The model under review builds one solid part; all positions refer to its coordinate system, in mm. Face numbers are marked on the shaded views. A direction names the side the tool comes from. Give positions to 0.01 mm unless a question says otherwise; leave off trailing zeros. Loops run counter-clockwise (first coordinate to the right, second up) from the corner with the lowest first, then second, coordinate; pieces in that order, holes last. Notation, with made-up numbers: M 61.25,45.25 L 101.25,45.25 A12 ccw 101.25,55.25 Z; hole C 13.25,22 d4. An arc over 180 degrees is marked long. Put each result on its own line as item: value. Start each with the question number.
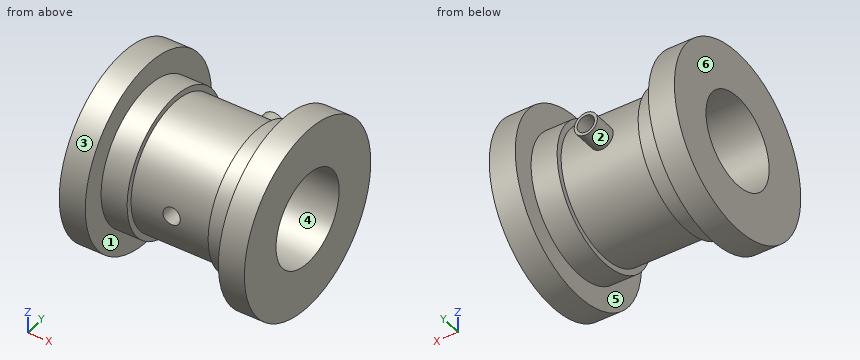
```python
from build123d import *

# Parameters (mm, degrees)
BOSS_EXTRUDE1_REACH      = 96.678
BOSS_EXTRUDE1_END_RADIUS = 22
SKETCH2_R                = 4
SKETCH3_R                = 3
CUT_EXTRUDE1_DEPTH       = 95.678403028


with BuildPart() as part:
    # Sketch1 → Revolve1 (revolve)
    with BuildSketch(Plane.XY, mode=Mode.PRIVATE) as revolve1_sk:
        Polygon((0, 16), (64, 16), (64, 32), (55, 32), (55, 24), (46, 24), (46, 22), (18, 22), (18, 24), (9, 24), (9, 32), (0, 32), align=None)
    revolve(revolve1_sk.sketch.rotate(Axis((0, 0, 0), (1, 0, 0)), 90), axis=Axis((0, 0, 0), (1, 0, 0)))

    # Boss-Extrude1: up to this cylinder (the profile starts outside it)
    boss_extrude1_end = Plane(origin=(32, 0, 0), z_dir=(-1, 0, 0)) * Cylinder(BOSS_EXTRUDE1_END_RADIUS, 238.356, mode=Mode.PRIVATE)
    # Sketch2 → Boss-Extrude1 (add, up to the surface)
    with BuildSketch(Plane(origin=(0, 30, 0), x_dir=(1, 0, 0), z_dir=(0, 1, 0)), mode=Mode.PRIVATE) as boss_extrude1_sk1:
        with Locations(Location((32, -1, 0), (0, 0, 270))):
            Circle(SKETCH2_R)
    boss_extrude1_tool1 = extrude(boss_extrude1_sk1.sketch, amount=-BOSS_EXTRUDE1_REACH, mode=Mode.PRIVATE) - boss_extrude1_end
    add(boss_extrude1_tool1.solids().sort_by_distance((32, 30, 1))[0])

    # Sketch3 → Cut-Extrude1 (cut, through all)
    with BuildSketch(Plane(origin=(0, 30, 0), x_dir=(1, 0, 0), z_dir=(0, 1, 0))):
        with Locations(Location((32, -1, 0), (0, 0, 270))):
            Circle(SKETCH3_R)
    extrude(amount=-CUT_EXTRUDE1_DEPTH, mode=Mode.SUBTRACT)


solid = part.part
```
Item 1: Clearance check with flat-ended pins moving along their axes: pin 1 Ø6.5 at (x, z) = (30.5, 0.5) entering from +Y; pin 2 Ø6 at (x, z) = (22.5, 7.5) entering from +Y; pin 3 Ø12 at (y, z) = (-6, 22) entering from -X; pin 4 Ø1.5 at (x, y) = (44, 4) entering from -Z. State where each tip first meets the part, or that it passes through.
Item 2: Consider section C-C, the plane z = -7. Write out the cut boundary in (x, y).
Item 3: To check wall thickness, follow L1, parallel to X at y = -17, z = -15; L2, parallel to X at y = 23, z = 1; L3, parallel to Z at x = 32, y = 25. State the ranges of each line that lie inside material, in increasing order. Write a range as [from, to].
Item 4: Draft analysis for pull direction X (two halves, no side actions). For the marked faces 4, 5 and 6, state which applies: +X half, -X half, draft (parallel to the pull), parting line (faces both ways), or undercut.
Item 5: Tool access review of the marked faces 1, 2 and 3: name each direction out of +Z, -Z, +X, -X, +Y, -Y from which nothing blocks a thin tool from reaching the whole face with its end or side.
Item 6: Consider section B-B, the plane x = 32. Write out the cut boundary in (y, z).
Item 7: Consider section A-A, the plane y = -11. Write out the cut boundary in (x, z), plus the area to 3 significant figures.
Item 8: Consider section D-D, the plane x = 23.5. Write out the cut boundary in (y, z).
Report:
1. pin 1: y = 30
1. pin 2: y = 21.53
1. pin 3: x = 0
1. pin 4: z = -21.76
2. outline: M 0,-31.22 L 9,-31.22 L 9,-22.96 L 18,-22.96 L 18,-20.86 L 46,-20.86 L 46,-22.96 L 55,-22.96 L 55,-31.22 L 64,-31.22 L 64,-14.39 L 0,-14.39 Z; M 0,14.39 L 64,14.39 L 64,31.22 L 55,31.22 L 55,22.96 L 46,22.96 L 46,20.86 L 18,20.86 L 18,22.96 L 9,22.96 L 9,31.22 L 0,31.22 Z
3. L1: [0, 18], [46, 64]
3. L2: [0, 18], [28, 29], [35, 36], [46, 64]
3. L3: [-3, -2], [4, 5]
4. face 4: draft
4. face 5: undercut
4. face 6: -X half
5. face 1: none
5. face 2: +Y
5. face 3: +X, -X
6. outline: M -21.91,-2 A22 ccw 21.79,-3 L 30,-3 L 30,-2 L 15.87,-2 A16 cw -15.87,-2 Z; M -21.63,4 L -15.49,4 A16 cw 15.49,4 L 30,4 L 30,5 L 21.42,5 A22 ccw Z
7. outline: M 0,-30.05 L 9,-30.05 L 9,-21.33 L 18,-21.33 L 18,-19.05 L 46,-19.05 L 46,-21.33 L 55,-21.33 L 55,-30.05 L 64,-30.05 L 64,-11.62 L 0,-11.62 Z; M 0,11.62 L 64,11.62 L 64,30.05 L 55,30.05 L 55,21.33 L 46,21.33 L 46,19.05 L 18,19.05 L 18,21.33 L 9,21.33 L 9,30.05 L 0,30.05 Z
7. area: 1,430 mm²
8. outline: C 0,0 d44; hole C 0,0 d32
